Input: part model. Units: mm. Frame: model coordinates. Face numbers are marked on the shaded views. A direction names the side the tool comes from. Give positions to 0.01 mm unless a question says otherwise; leave off trailing zeros. Loops run counter-clockwise (first coordinate to the right, second up) from the corner with the lowest first, then second, coordinate; pieces in that order, holes last. Notation, with made-up numbers: M 0,65 L 4,65 A17 ccw 4,83 Z; hole C 29.25,84 d1. An arc over 180 degrees is marked long. One line per item, written item: value. Start each with the question number.
(1) Access query for the marked faces 4, 5 and 6. Directions: +Z, -Z, +X, -X, +Y, -Y. A direction counts if a zero-diameter tool reaches every point of the face in a straight line with its end or side. Return the directions, or none.
(2) Section B-B on y = 17.6. Output: boundary loops of the cut face in (x, z).
(3) Section A-A on z = 27.88. Output: boundary loops of the cut face in (x, y).
(4) Pin query (flat end, axial travel): P1, Ø10, axis at x = 48, z = 26.5, coming from the -Y side; P2, Ø1.8, axis at y = 2.5, z = 22, coming from the +X side; P3, Ø12, axis at y = 31.5, z = 14.5, coming from the +X side; P4, Ø1.6, axis at x = 27.996, y = 2.8, coming from the -Z side. Return the tip coordinate at first contact, or that it passes through.
(5) Pull-direction query (Z, two-part tool) for the marked faces 1, 2 and 3; classes: released by +Z, released by -Z, zero draft, split by the parting line, or undercut.
(6) Ray query, line 1 along Y through (x, z) = (3.9, 27.88); line 2 along X through (y, z) = (2, 1); line 3 along X through (y, z) = (3.5, 2). Return the intervals inside material, ascending. Write a range as from..to.
(7) Section D-D on y = 2.8. State how many separate pieces and enclosed holes the cut face has, plus the area to 3 significant figures.
(8) Section C-C on x = 39.5. Output: boundary loops of the cut face in (y, z), plus the area to 3 significant figures.
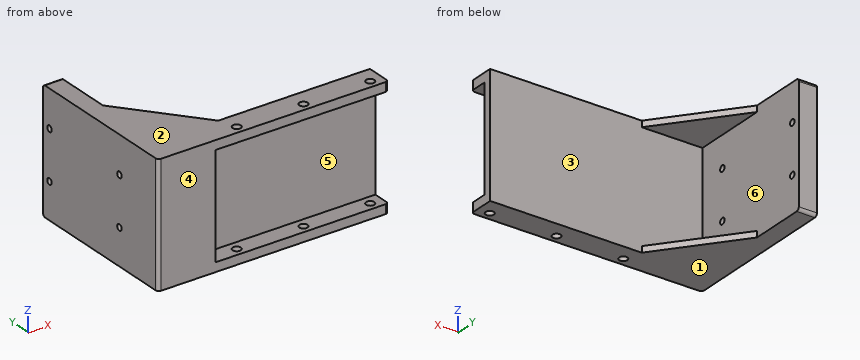
```python
from build123d import *

# Parameters (mm, degrees)
BOSS_EXTRUDE1_DEPTH = 40.1
SKETCH3_R           = 1.35
CUT_EXTRUDE2_DEPTH  = 50.8
SKETCH4_R           = 1.016
CUT_EXTRUDE3_DEPTH  = 50.8
SKETCH6_W           = 62.086073973
SKETCH6_H           = 34.1
CUT_EXTRUDE4_DEPTH  = 6
BOSS_EXTRUDE5_DEPTH = 2
FILLET1_R           = 1


with BuildPart() as part:
    # Sketch1 → Boss-Extrude1 (new body)
    with BuildSketch(Plane.XY):
        Polygon((0, 0), (0, 52.578), (6, 52.578), (6, 8.5), (76, 8.5), (76, 0), align=None)
    extrude(amount=BOSS_EXTRUDE1_DEPTH)

    # Sketch3 → Cut-Extrude2 (cut)
    with BuildSketch(Plane.XY.offset(40.1)):
        with Locations((27.996, 2.8)):
            Circle(SKETCH3_R)
        with Locations((49.996, 2.8)):
            Circle(SKETCH3_R)
        with Locations((71.996, 2.8)):
            Circle(SKETCH3_R)
    extrude(amount=-CUT_EXTRUDE2_DEPTH, mode=Mode.SUBTRACT)

    # Sketch4 → Cut-Extrude3 (cut)
    with BuildSketch(Plane.ZY):
        with Locations((27.88, 17.6)):
            Circle(SKETCH4_R)
        with Locations(Location((11.88, 17.6, 0), (0, 0, 270))):
            Circle(SKETCH4_R)
        with Locations((27.88, 49.6)):
            Circle(SKETCH4_R)
        with Locations(Location((11.88, 49.6, 0), (0, 0, 270))):
            Circle(SKETCH4_R)
    extrude(amount=-CUT_EXTRUDE3_DEPTH, mode=Mode.SUBTRACT)

    # Sketch6 → Cut-Extrude4 (cut)
    with BuildSketch(Plane.XZ):
        with Locations((50.043036987, 20.05)):
            Rectangle(SKETCH6_W, SKETCH6_H)
    extrude(amount=-CUT_EXTRUDE4_DEPTH, mode=Mode.SUBTRACT)

    # Sketch16 → Boss-Extrude5 (add)
    with BuildSketch(Plane.XY.offset(40.1)):
        Polygon((6, 8.5), (26, 8.5), (6, 33.5), align=None)
    boss_extrude5 = extrude(amount=-BOSS_EXTRUDE5_DEPTH)

    # Mirror2: Boss-Extrude5 across plane
    add(boss_extrude5.mirror(Plane(origin=(0, 0, 20.05), x_dir=(1, 0, 0), z_dir=(0, 0, -1))))

    # Fillet1
    fillet1_edges = [part.edges().sort_by_distance(p)[0] for p in [
        (0, 0, 20.05),
        (76, 0, 38.6),
        (3, 52.578, 40.1),
        (76, 0, 1.5),
        (3, 52.578, 0),
    ]]
    fillet(fillet1_edges, radius=FILLET1_R)


solid = part.part
```
Output values:
1. face 4: +Z, -Z, +X, -X, -Y
1. face 5: +X, -Y
1. face 6: +X, +Y
2. outline: M 0,0 L 18.72,0 L 18.72,2 L 6,2 L 6,10.86 L 0,10.86 Z; M 0,12.9 L 6,12.9 L 6,26.86 L 0,26.86 Z; M 0,28.9 L 6,28.9 L 6,38.1 L 18.72,38.1 L 18.72,40.1 L 0,40.1 Z
3. outline: M 0,1 A1 ccw 1,0 L 19,0 L 19,6 L 76,6 L 76,8.5 L 6,8.5 L 6,16.58 L 0,16.58 Z; M 0,18.62 L 6,18.62 L 6,48.58 L 0,48.58 Z; M 0,50.62 L 6,50.62 L 6,52.58 L 0,52.58 Z
4. P1: stops at y = 6
4. P2: stops at x = 19
4. P3: stops at x = 6
4. P4: passes through
5. face 1: released by -Z
5. face 2: released by +Z
5. face 3: undercut
6. line 1: y = 0..16.58, 18.62..48.58, 50.62..52.58
6. line 2: x = 0..26.91, 29.08..48.91, 51.08..70.91, 73.08..76
6. line 3: x = 0..26.84, 29.15..48.84, 51.15..70.84, 73.15..76
7. separate pieces: 7
7. enclosed holes: 0
7. area: 1,060 mm²
8. outline: M 0,0 L 8.5,0 L 8.5,40.1 L 0,40.1 L 0,37.1 L 6,37.1 L 6,3 L 0,3 Z
8. area: 136 mm²
